Source: CAD feature listing. Evaluate the final solid. Frame: model axes, mm. A direction names the side the tool comes from. Give positions to 0.01 mm unless a question says otherwise; leave off trailing zeros. Order: outer loops, then holes, each group sorted by start corner. A loop starts at its lowest first (then second) coordinate and runs counter-clockwise, first axis right, second up. Notation, with made-up numbers: M 72,1 L 123,1 A18 cw 123,13 Z; hole C -37,-24.5 d7. An arc over 180 degrees is marked long. One line per question, with ' | ' between items. Start each with the question number.
from build123d import *

# Parameters (mm, degrees)
F0_W     = 0.75
F0_H     = 6
F1_DEPTH = 10
F2_R     = 1.6
F3_DEPTH = 25
F4_DEPTH = 1
F5_R     = 1
F6_R     = 0.5


with BuildPart() as f1:
    # F0 (on Top) → F1 (new body)
    with BuildSketch(Plane.XY):
        with Locations((-0.375, 0)):
            Rectangle(F0_W, F0_H)
        Polygon((0, 8), (0, 3), (0, -3), (0, -8), (5.25, -8), (5.25, 8), align=None)
    extrude(amount=F1_DEPTH)

    # F2 (on face) → F3 (cut)
    with BuildSketch(Plane.YZ.offset(5.25)):
        with Locations((0, 5)):
            Circle(F2_R)
    extrude(amount=-F3_DEPTH, mode=Mode.SUBTRACT)

    # F2 (on face) → F4 (join)
    with BuildSketch(Plane.YZ.offset(5.25)):
        with BuildLine():
            ThreePointArc((-3.25, 5), (0, 8.25), (3.25, 5))
            Line((3.25, 5), (3.25, 10))
            Line((3.25, 10), (-3.25, 10))
            Line((-3.25, 10), (-3.25, 5))
        make_face()
        with BuildLine():
            ThreePointArc((-3.25, 5), (0, 1.75), (3.25, 5))
            ThreePointArc((3.25, 5), (0, 8.25), (-3.25, 5))
        make_face()
        with Locations((0, 5)):
            Circle(F2_R, mode=Mode.SUBTRACT)
        with BuildLine():
            Line((3.25, 0), (3.25, 5))
            ThreePointArc((3.25, 5), (0, 1.75), (-3.25, 5))
            Line((-3.25, 5), (-3.25, 0))
            Line((-3.25, 0), (3.25, 0))
        make_face()
    extrude(amount=F4_DEPTH)

    # F5
    f5_edges = [f1.edges().sort_by_distance(p)[0] for p in [
        (5.25, -8, 5),
        (5.25, 8, 5),
    ]]
    fillet(f5_edges, radius=F5_R)

    # F6
    f6_edges = [f1.edges().sort_by_distance(p)[0] for p in [
        (-0.75, -3, 5),
        (-0.75, 3, 5),
    ]]
    fillet(f6_edges, radius=F6_R)


solid = f1.part
Item 1: Cut plane C-C on z = 2.25. Return the cut outline in (x, y).
Item 2: Cut plane A-A on z = 5. Return the cut outline in (x, y), and give its area (3 significant figures).
Item 3: Line query: line 1 (Z direction, x = 5.85, y = 0); line 2 (X direction, y = 5.5, z = 9); line 3 (Y direction, x = 0.5, z = 6.25). Output: solid intervals per line, ascending.
Item 4: Cut plane B-B on y = 0. Return the cut outline in (x, z), and give its area (3 significant figures).
Item 5: Pin query (flat end, axial travel): pin 1 Ø4 at (y, z) = (6, 4) entering from +X; pin 2 Ø2.5 at (y, z) = (5, 5) entering from -X; pin 3 Ø1.1 at (x, z) = (6, 7.5) entering from +Y. Return the tip coordinate at first contact, or that it passes through.
Item 6: Reachability of faces 1 (the flat face through (0, -5, 5)), 2 (the flat face through (5.25, 5, 5)), 3 (the flat face through (6, -3.25, 5)) from +Z, -Z, +X, -X, +Y, -Y: full face, straight path, thin tool, end or side. Return the list, or none.
Item 7: Cut plane D-D on x = 0.75. Return the cut outline in (y, z).
Results are:
1) outline: M -0.75,-2.5 A0.5 ccw -0.25,-3 L 0,-3 L 0,-8 L 4.25,-8 A1 ccw 5.25,-7 L 5.25,-3.25 L 6.25,-3.25 L 6.25,3.25 L 5.25,3.25 L 5.25,7 A1 ccw 4.25,8 L 0,8 L 0,3 L -0.25,3 A0.5 ccw -0.75,2.5 Z
2) outline: M -0.75,-2.5 A0.5 ccw -0.25,-3 L 0,-3 L 0,-8 L 4.25,-8 A1 ccw 5.25,-7 L 5.25,-3.25 L 6.25,-3.25 L 6.25,-1.6 L -0.75,-1.6 Z; M -0.75,1.6 L 6.25,1.6 L 6.25,3.25 L 5.25,3.25 L 5.25,7 A1 ccw 4.25,8 L 0,8 L 0,3 L -0.25,3 A0.5 ccw -0.75,2.5 Z | area: 72.1 mm2
3) line 1: z = 0 to 3.4, 6.6 to 10 | line 2: x = 0 to 5.25 | line 3: y = -8 to -1, 1 to 8
4) outline: M -0.75,0 L 6.25,0 L 6.25,3.4 L -0.75,3.4 Z; M -0.75,6.6 L 6.25,6.6 L 6.25,10 L -0.75,10 Z | area: 47.6 mm2
5) pin 1: stops at x = 5.25 | pin 2: stops at x = 0 | pin 3: stops at y = 3.25
6) face 1: +Z, -Z, -X, -Y | face 2: +Z, -Z, +X, +Y | face 3: +Z, -Z, +X, -Y
7) outline: M -8,0 L 8,0 L 8,10 L -8,10 Z; hole C 0,5 d3.2
